For this review, take the finished solid that the model builds, in its own axes (mm). A direction names the side the tool comes from. Round coordinates to 2 decimals unless told otherwise and drop trailing zeros. Write each loop counter-clockwise with the first axis right and the second up, starting at its lowest first coordinate (ties: lowest second). Pieces come first, ordered by that corner, then holes. Notation, with made-up numbers: M -23,-11.5 L -12,-11.5 A19 cw -12,12.5 Z; hole C 13.25,69 d4. An arc over 180 degrees is marked long. Answer in a Markdown table with one row per item.
```python
from build123d import *

# Parameters (mm, degrees)
F0_R     = 20
F1_DEPTH = 15
F2_R     = 17.5
F2_R_2   = 2.5
F3_DEPTH = 6
F4_R     = 1.5
F5_DEPTH = 25
F6_R     = 17.5
F6_R_2   = 2.5
F7_DEPTH = 6
F8_DEPTH = 25


with BuildPart() as f1:
    # F0 (on Right) → F1 (new body)
    with BuildSketch(Plane.YZ):
        Circle(F0_R)
    extrude(amount=F1_DEPTH)

    # F2 (on face) → F3 (cut)
    with BuildSketch(Plane.YZ.offset(15)):
        Circle(F2_R)
        Circle(F2_R_2, mode=Mode.SUBTRACT)
    extrude(amount=-F3_DEPTH, mode=Mode.SUBTRACT)

    # F4 (on face) → F5 (cut)
    with BuildSketch(Plane.YZ.offset(15)):
        Circle(F4_R)
    extrude(amount=-F5_DEPTH, mode=Mode.SUBTRACT)

    # F6 (on face) → F7 (cut)
    with BuildSketch(Plane(origin=(0, 0, 0), x_dir=(0, -1, 0), z_dir=(-1, 0, 0))):
        Circle(F6_R)
        Circle(F6_R_2, mode=Mode.SUBTRACT)
    extrude(amount=-F7_DEPTH, mode=Mode.SUBTRACT)

    # F8 (cut): a face of the model
    f8_faces = [f1.faces().sort_by_distance(p)[0] for p in [
        (15, -19.4343145751, 0),
    ]]
    extrude(f8_faces, amount=-F8_DEPTH, mode=Mode.SUBTRACT)


solid = f1.part
```
Q1. Take a section at C-C (x = 13.5). State the section outline as (y, z) points, then the cut area to 3 significant figures.
Found:
| item | result |
|---|---|
| outline | C 0,0 d5; hole C 0,0 d3 |
| area | 12.6 mm² |
Q2. For probe 1 along Z at (x, y) = (10.5, 0); probe 2 along Z at (x, y) = (7, 0); probe 3 along X at (y, z) = (-6, 2), list the stretches that pass through material, from the lowest coordinate up.
Found:
| item | result |
|---|---|
| probe 1 | -2.5 to -1.5, 1.5 to 2.5 |
| probe 2 | -17.5 to -1.5, 1.5 to 17.5 |
| probe 3 | 6 to 9 |
Q3. Take a section at A-A (z = 0). State the section outline as (x, y) points.
Found:
| item | result |
|---|---|
| outline | M 0,-2.5 L 6,-2.5 L 6,-17.5 L 9,-17.5 L 9,-2.5 L 15,-2.5 L 15,-1.5 L 0,-1.5 Z; M 0,1.5 L 15,1.5 L 15,2.5 L 9,2.5 L 9,17.5 L 6,17.5 L 6,2.5 L 0,2.5 Z |
Q4. Take a section at D-D (y = -5.5). State the section outline as (x, z) points.
Found:
| item | result |
|---|---|
| outline | M 6,-16.61 L 9,-16.61 L 9,16.61 L 6,16.61 Z |
Q5. Mouldability with a two-part tool opening along Z and no side actions: class faces 1 (the face through (15, 0, -2)), 2 (the face through (7.6, -1.5, 0.07)), 3 (the face through (12.04, -0.54, -2.44)) as +Z half, -Z half, draft (parallel to the pull), parting line (faces both ways), or undercut.
Found:
| item | result |
|---|---|
| face 1 | draft |
| face 2 | undercut |
| face 3 | parting line |
Q6. Machinability: for faces 4 (the face through (7.521, -13.887, -10.648)), 5 (the face through (2.96, 0.54, -2.44)), which of the approach directions +Z, -Z, +X, -X, +Y, -Y give a long, thin tool a straight path to every point of the face, cutting with its end or side? Answer none if there is none.
Found:
| item | result |
|---|---|
| face 4 | +X, -X |
| face 5 | -X |
Q7. Insertion check: P1, Ø3, axis at y = 6, z = -7.5, coming from the -X side; P2, Ø1.5, axis at x = 6.5, z = 5.5, coming from the -Y side. Each pin has a flat end and moves straight along its axis. Give the tip position at first contact, or say it passes through.
Found:
| item | result |
|---|---|
| P1 | x = 6 |
| P2 | y = -16.84 |
